Here's how the part is built. I have some questions about the finished solid (model axes, mm). A direction names the side the tool comes from. Round coordinates to 2 decimals unless told otherwise and drop trailing zeros. Loops run counter-clockwise (first coordinate to the right, second up) from the corner with the lowest first, then second, coordinate; pieces in that order, holes last. Notation, with made-up numbers: M -25.5,-23 L 27.5,-23 A15 cw 27.5,-1 Z; hole C -40,67.5 d1. An arc over 180 degrees is marked long. Answer as a JSON object with one key per item and string values.
from build123d import *

# Parameters (mm, degrees)
F0_W     = 79
F0_H     = 37.4
F1_DEPTH = 9
F2_W     = 62
F2_H     = 26
F3_DEPTH = 0.3
F4_R     = 1
F5_W     = 1
F5_H     = 1
F6_DEPTH = 25.4
F7_W     = 87
F7_H     = 60
F8_DEPTH = 1.6
F10_D    = 2.5
F12_D    = 1


with BuildPart() as f1:
    # F0 (on Front) → F1 (new body)
    with BuildSketch(Plane.XZ):
        Rectangle(F0_W, F0_H)
    extrude(amount=F1_DEPTH)

    # F2 (on face) → F3 (cut)
    with BuildSketch(Plane.XZ.offset(9)):
        Rectangle(F2_W, F2_H)
    extrude(amount=-F3_DEPTH, mode=Mode.SUBTRACT)

    # F4
    f4_edges = [f1.edges().sort_by_distance(p)[0] for p in [
        (-31, -8.85, 13),
        (31, -8.85, 13),
        (31, -8.85, -13),
        (-31, -8.85, -13),
    ]]
    fillet(f4_edges, radius=F4_R)

    # F5 (on face) → F6 (cut)
    with BuildSketch(Plane.XZ.offset(9)):
        with Locations((-39, -18.2)):
            Rectangle(F5_W, F5_H)
        with Locations((39, -18.2)):
            Rectangle(F5_W, F5_H)
        with Locations((39, 18.2)):
            Rectangle(F5_W, F5_H)
        with Locations((-39, 18.2)):
            Rectangle(F5_W, F5_H)
    extrude(amount=-F6_DEPTH, mode=Mode.SUBTRACT)

    # F7 (on face) → F8 (join)
    with BuildSketch(Plane(origin=(0, 0, 0), x_dir=(-1, 0, 0), z_dir=(0, 1, 0))):
        Rectangle(F7_W, F7_H)
    extrude(amount=F8_DEPTH)

    # F10 (through all)
    with Locations(Plane.XZ):
        with Locations((-41, 27.5), (-41, -27.5), (41, 27.5), (41, -27.5)):
            Hole(F10_D / 2)

    # F12 (through all)
    with Locations(Plane.XZ):
        with Locations((-33.5, 27.5), (-30.96, 27.5), (-28.42, 27.5), (-25.88, 27.5), (-23.34, 27.5), (-20.8, 27.5), (-18.26, 27.5), (-15.72, 27.5), (-13.18, 27.5), (-10.64, 27.5), (-8.1, 27.5), (-5.56, 27.5), (-3.02, 27.5), (-0.48, 27.5), (2.06, 27.5), (4.6, 27.5)):
            Hole(F12_D / 2)


solid = f1.part
Item 1: I want a section at D-D, the plane z = 21.5. Please give me the cut outline in (x, y).
Resolved:
{"outline": "M -43.5,0 L 43.5,0 L 43.5,1.6 L -43.5,1.6 Z"}
Item 2: I want a section at B-B, the plane z = 9. Please give me the cut outline in (x, y).
Resolved:
{"outline": "M -43.5,0 L -39.5,0 L -39.5,-9 L -31,-9 L -31,-8.7 L 31,-8.7 L 31,-9 L 39.5,-9 L 39.5,0 L 43.5,0 L 43.5,1.6 L -43.5,1.6 Z"}
Item 3: On a 3-axis mill with a long thin cutter (end or side, diameter ignored), from which of +Z, -Z, +X, -X, +Y, -Y can I reach the whole of each face in a straight line? I mean faces 4 (the face through (-1, -4, -18.7)), 5 (the face through (0, -8.7, 0)), 6 (the face through (39.5, -4, 0)), 7 (the face through (-1, -4, 18.7)). Say none if no direction works.
Resolved:
{"face 4": "-Z, +X, -X, -Y", "face 5": "-Y", "face 6": "+Z, -Z, +X, -Y", "face 7": "+Z, +X, -X, -Y"}
Item 4: I want a section at C-C, the plane y = -1. Please give me the cut outline in (x, z).
Resolved:
{"outline": "M -39.5,-17.7 L -38.5,-17.7 L -38.5,-18.7 L 38.5,-18.7 L 38.5,-17.7 L 39.5,-17.7 L 39.5,17.7 L 38.5,17.7 L 38.5,18.7 L -38.5,18.7 L -38.5,17.7 L -39.5,17.7 Z"}
Item 5: Please list where these lines run through material, in increasing order: probe 1 along Z at (x, y) = (-0.48, 0.9); probe 2 along Z at (x, y) = (4, -3); probe 3 along Y at (x, z) = (13, -21.5). Write a range as from..to.
Resolved:
{"probe 1": "-30..27, 28..30", "probe 2": "-18.7..18.7", "probe 3": "0..1.6"}
Item 6: I want a section at A-A, the plane x = -41. Please give me the cut outline in (y, z).
Resolved:
{"outline": "M 0,-30 L 1.6,-30 L 1.6,-28.75 L 0,-28.75 Z; M 0,-26.25 L 1.6,-26.25 L 1.6,26.25 L 0,26.25 Z; M 0,28.75 L 1.6,28.75 L 1.6,30 L 0,30 Z"}
Item 7: If we mould it in two halves opening along X, with no side actions, what happens to faces 1 (the face through (42.25, 0.81, 27.55)), 2 (the face through (1, 1, 30)), 3 (the face through (-39.5, -4, 0))? For each: pulls with the +X half, pulls with the -X half, needs draft (parallel to the pull), parting line crosses it, or undercut.
Resolved:
{"face 1": "undercut", "face 2": "needs draft", "face 3": "pulls with the -X half"}
Item 8: I'm going to push flat-ended pins straight in: pin 1 Ø8 at (x, z) = (-1, -6) entering from -Y; pin 2 Ø4 at (y, z) = (-6.5, 12) entering from +X; pin 3 Ø4 at (x, z) = (-41, -27.5) entering from +Y; pin 4 Ø2.5 at (x, y) = (-18.5, -4.5) entering from -Z. Where does each tip first touch, or does it pass through?
Resolved:
{"pin 1": "y = -8.7", "pin 2": "x = 39.5", "pin 3": "y = 1.6", "pin 4": "z = -18.7"}
